Could you check a few things on this model? Use its own coordinates, in mm. Face numbers are marked on the shaded views. A direction names the side the tool comes from. Give positions to 0.01 mm unless a question says otherwise; leave off trailing zeros. Loops run counter-clockwise (first coordinate to the right, second up) from the corner with the lowest first, then second, coordinate; pieces in that order, holes last. Notation, with made-up numbers: (87.5, 81) - (112.5, 81) arc R13 cw to (112.5, 103) - close; hole circle Ø5 at (18, 16.5). An arc over 180 degrees is marked (long way). One line per item, written item: value. Start each with the question number.
Q1. I want a section at A-A (x = -3.5). Please give me the cut outline in (y, z).
Q2. I want a section at C-C (y = -7). Please give me the cut outline in (x, z), then the cut area to 3 significant figures.
Q3. I want a section at B-B (x = 0). Please give me the cut outline in (y, z), then the cut area to 3 significant figures.
Q4. If we mould it in two halves opening along Y, with no side actions, what happens to the marked faces 5, 6 and 7? For each: released by +Y, released by -Y, zero draft, split by the parting line, or undercut.
Q5. I want a section at D-D (z = 7.75). Please give me the cut outline in (x, y).
Q6. For the marked faces 1, 2, 3 and 4, which set-ups out of +Z, -Z, +X, -X, +Y, -Y let a thin tool reach every point of the face, with its end or its side?
Q7. If I drill on line 1 (Y direction, x = -4.75, z = 3); line 2 (Z direction, x = 3, y = -6); line 3 (Y direction, x = -7.5, z = 5.5), over which ranges is the centre line in solid material (lowest first)? Write a range as from..to.
Q8. I'm going to push flat-ended pins straight in: P1, Ø7, axis at x = 4.953, y = -24.638, coming from the +Z side; P2, Ø7.5, axis at x = -0.5, y = 23.5, coming from the +Z side; P3, Ø1.5, axis at x = 7.5, z = 6, coming from the -Y side. Where does each tip first touch, or does it pass through?
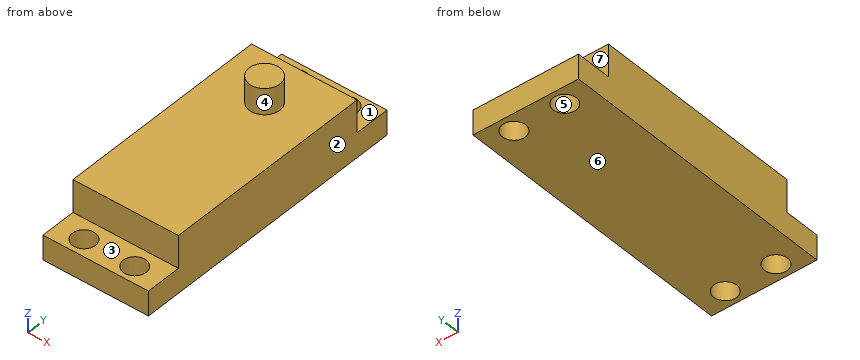
```python
from build123d import *

# Parameters (mm, degrees)
SKETCH1_W             = 20.574
SKETCH1_H             = 55.626
BOSS_EXTRUDE1_DEPTH   = 11.176
SKETCH2_R             = 2.9845
BOSS_EXTRUDE2_DEPTH   = 5.08
F_8_CLEARANCE_HOLE1_D = 4.4958
MIRROR2_COPY_1_D      = 4.4958
SKETCH6_W             = 6.35
SKETCH6_H             = 6.985
CUT_EXTRUDE1_DEPTH    = 21.574


with BuildPart() as part:
    # Sketch1 → Boss-Extrude1 (new body)
    with BuildSketch(Plane.XY):
        Rectangle(SKETCH1_W, SKETCH1_H)
    extrude(amount=BOSS_EXTRUDE1_DEPTH)

    # Sketch2 → Boss-Extrude2 (add)
    with BuildSketch(Plane.XY.offset(11.176)):
        with Locations((0, 11.557)):
            Circle(SKETCH2_R)
    extrude(amount=BOSS_EXTRUDE2_DEPTH)

    # #8 Clearance Hole1 (through all)
    with Locations(Plane(origin=(0, 0, 0), x_dir=(-1, 0, 0), z_dir=(0, 0, -1))):
        with Locations((4.953, 24.638)):
            f_8_clearance_hole1 = Hole(F_8_CLEARANCE_HOLE1_D / 2)

    # Mirror1: #8 Clearance Hole1 across plane
    add(f_8_clearance_hole1.mirror(Plane(origin=(0, 0, 0), x_dir=(0, 0, 1), z_dir=(1, 0, 0))), mode=Mode.SUBTRACT)

    # Mirror2: #8 Clearance Hole1 across plane
    add(f_8_clearance_hole1.mirror(Plane.ZX), mode=Mode.SUBTRACT)

    # Mirror2 copy 1 (through all)
    with Locations(Plane(origin=(0, 0, 0), x_dir=(1, 0, 0), z_dir=(0, 0, -1))):
        with Locations((4.953, 24.638)):
            Hole(MIRROR2_COPY_1_D / 2)

    # Sketch6 → Cut-Extrude1 (cut, through all)
    with BuildSketch(Plane.ZY.offset(10.287)):
        with Locations((8.001, -24.3205)):
            Rectangle(SKETCH6_W, SKETCH6_H)
        with Locations((8.001, 24.3205)):
            Rectangle(SKETCH6_W, SKETCH6_H)
    extrude(amount=-CUT_EXTRUDE1_DEPTH, mode=Mode.SUBTRACT)


solid = part.part
```
Worked answers:
1. outline: (-27.81, 0) - (-26.35, 0) - (-26.35, 4.83) - (-27.81, 4.83) - close; (-22.92, 0) - (22.92, 0) - (22.92, 4.83) - (20.83, 4.83) - (20.83, 11.18) - (-20.83, 11.18) - (-20.83, 4.83) - (-22.92, 4.83) - close; (26.35, 0) - (27.81, 0) - (27.81, 4.83) - (26.35, 4.83) - close
2. outline: (-10.29, 0) - (10.29, 0) - (10.29, 11.18) - (-10.29, 11.18) - close
2. area: 230 mm²
3. outline: (-27.81, 0) - (27.81, 0) - (27.81, 4.83) - (20.83, 4.83) - (20.83, 11.18) - (14.54, 11.18) - (14.54, 16.26) - (8.57, 16.26) - (8.57, 11.18) - (-20.83, 11.18) - (-20.83, 4.83) - (-27.81, 4.83) - close
3. area: 563 mm²
4. face 5: undercut
4. face 6: zero draft
4. face 7: released by +Y
5. outline: (-10.29, -20.83) - (10.29, -20.83) - (10.29, 20.83) - (-10.29, 20.83) - close
6. face 1: +Z, +X, -X, +Y
6. face 2: +Z, -Z, +X, +Y, -Y
6. face 3: +Z, +X, -X, -Y
6. face 4: +Z
7. line 1: y = -27.81..-26.88, -22.4..22.4, 26.88..27.81
7. line 2: z = 0..11.18
7. line 3: y = -20.83..20.83
8. P1: stops at z = 4.83
8. P2: stops at z = 11.18
8. P3: stops at y = -20.83
